Work out the finished part from the listing and answer in its coordinate system (mm). Coordinates: 2 decimals unless noted, no trailing zeros. Write each loop counter-clockwise with the first axis right and the second up, starting at its lowest first coordinate (ties: lowest second). Pieces come first, ordered by that corner, then holes. Notation, with made-up numbers: (55, 46) - (86, 46) arc R24 ccw to (86, 83) - close; hole circle Ø7 at (42, -1). An arc over 180 degrees is marked (long way). Use CSV: the item, a comma, the result in double quotes. Start each with the question number.
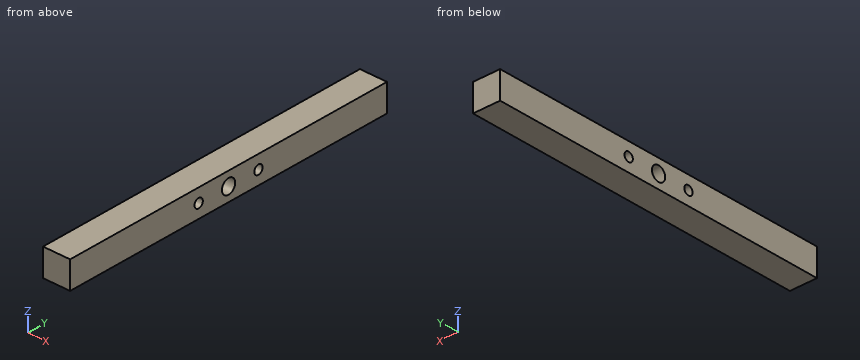
from build123d import *

# Parameters (mm, degrees)
SKETCH_1_W          = 15
SKETCH_1_H          = 15
EXTRUDE_1_DEPTH     = 190.88
SKETCH_2_R          = 4
SKETCH_2_R_2        = 2.5
CUT_EXTRUDE_1_DEPTH = 192.615303147


with BuildPart() as part:
    # 草图1 → 凸台-拉伸1 (new body)
    with BuildSketch(Plane(origin=(0, 0, 0), x_dir=(1, 0, 0), z_dir=(0, 1, 0))):
        Rectangle(SKETCH_1_W, SKETCH_1_H)
    extrude(amount=EXTRUDE_1_DEPTH)

    # 草图2 → 切除-拉伸1 (cut, through all)
    with BuildSketch(Plane(origin=(7.5, 0, 0), x_dir=(0, 0, -1), z_dir=(1, 0, 0))):
        with Locations((0, 95.44)):
            Circle(SKETCH_2_R)
        with Locations((0, 113.44)):
            Circle(SKETCH_2_R_2)
        with Locations((0, 77.44)):
            Circle(SKETCH_2_R_2)
    extrude(amount=-CUT_EXTRUDE_1_DEPTH, mode=Mode.SUBTRACT)


solid = part.part
Item 1: Straight lines are drawn through the part: probe 1 along Y at (x, z) = (-3.5, 0); probe 2 along Y at (x, z) = (-2.25, -2.25); probe 3 along Y at (x, z) = (-2, -3). For each, find the intervals that lie inside material, in ascending order. Write a range as [from, to].
Item 2: A cutting plane is placed at C-C (x = -5.5). Determine the outline of the cut face in (y, z).
Item 3: A cutting plane is placed at A-A (y = 95.44). Determine the outline of the cut face in (x, z), then the cut area to 3 significant figures.
Item 4: A cutting plane is placed at B-B (z = 0). Determine the outline of the cut face in (x, y).
Calculated:
1,probe 1,"y = [0, 74.94], [79.94, 91.44], [99.44, 110.94], [115.94, 190.88]"
1,probe 2,"y = [0, 76.35], [78.53, 92.13], [98.75, 112.35], [114.53, 190.88]"
1,probe 3,"y = [0, 92.79], [98.09, 190.88]"
2,outline,"(0, -7.5) - (190.88, -7.5) - (190.88, 7.5) - (0, 7.5) - close; hole circle Ø5 at (77.44, 0); hole circle Ø8 at (95.44, 0); hole circle Ø5 at (113.44, 0)"
3,outline,"(-7.5, -7.5) - (7.5, -7.5) - (7.5, -4) - (-7.5, -4) - close; (-7.5, 4) - (7.5, 4) - (7.5, 7.5) - (-7.5, 7.5) - close"
3,area,"105 mm²"
4,outline,"(-7.5, 0) - (7.5, 0) - (7.5, 74.94) - (-7.5, 74.94) - close; (-7.5, 79.94) - (7.5, 79.94) - (7.5, 91.44) - (-7.5, 91.44) - close; (-7.5, 99.44) - (7.5, 99.44) - (7.5, 110.94) - (-7.5, 110.94) - close; (-7.5, 115.94) - (7.5, 115.94) - (7.5, 190.88) - (-7.5, 190.88) - close"
